Read the model definition and answer for the solid it produces. Units are mm, in the model's axes. Coordinates: 2 decimals unless noted, no trailing zeros. Write each loop counter-clockwise with the first axis right and the second up, starting at its lowest first coordinate (ties: lowest second). Pieces come first, ordered by that corner, then holes. Notation, with made-up numbers: M -32,0 L -19,0 A33 cw -19,29 Z; hole C 78.5,-14 d1. An arc over 180 degrees is marked long. Write item = value, one per line.
from build123d import *

# Parameters (mm, degrees)
BOSS_EXTRUDE2_DEPTH     = 4
SKETCH1_5_R             = 3
CUT_EXTRUDE3_DEPTH      = 54
SKETCH1_6_R             = 3
CUT_EXTRUDE4_DEPTH      = 35
CUT_EXTRUDE6_DEPTH      = 1.3
CUT_EXTRUDE6_DEPTH_BACK = 1.3


with BuildPart() as part:
    # Sketch1 → Boss-Extrude2 (new body)
    with BuildSketch(Plane(origin=(0, 0, 0), x_dir=(1, 0, 0), z_dir=(0, 1, 0))):
        with BuildLine():
            Line((-71.648984849, 27.5), (-138.40789612, 27.5))
            ThreePointArc((-138.40789612, 27.5), (-165.710949902, 25.175282852), (-192.40789612, 19))
            ThreePointArc((-192.40789612, 19), (-189.370573735, 12.036157899), (-188.40789612, 4.5))
            Line((-188.40789612, 4.5), (-120.40789612, 4.5))
            ThreePointArc((-120.40789612, 4.5), (-115.90789612, 0), (-120.40789612, -4.5))
            Line((-120.40789612, -4.5), (-188.40789612, -4.5))
            ThreePointArc((-188.40789612, -4.5), (-189.370573735, -12.036157899), (-192.40789612, -19))
            ThreePointArc((-192.40789612, -19), (-165.710949902, -25.175282852), (-138.40789612, -27.5))
            Line((-138.40789612, -27.5), (-71.648984849, -27.5))
            ThreePointArc((-71.648984849, -27.5), (65.101994969, -27.347428228), (201.798926373, -23.5))
            ThreePointArc((201.798926373, -23.5), (225.298926373, 0), (201.798926373, 23.5))
            ThreePointArc((201.798926373, 23.5), (65.101994969, 27.347428228), (-71.648984849, 27.5))
        make_face()
    extrude(amount=BOSS_EXTRUDE2_DEPTH)

    # Sketch1_5 → Cut-Extrude3 (cut)
    with BuildSketch(Plane(origin=(0, 0, 0), x_dir=(1, 0, 0), z_dir=(0, 1, 0))):
        with Locations((160.298926373, 0)):
            Circle(SKETCH1_5_R)
        with Locations((195.298926373, 0)):
            Circle(SKETCH1_5_R)
        with Locations((202.298926373, 7)):
            Circle(SKETCH1_5_R)
        with Locations((209.298926373, 0)):
            Circle(SKETCH1_5_R)
        with Locations((202.298926373, -7)):
            Circle(SKETCH1_5_R)
        with Locations((-169.40789612, -13.5)):
            Circle(SKETCH1_5_R)
    extrude(amount=CUT_EXTRUDE3_DEPTH, mode=Mode.SUBTRACT)

    # Sketch1_6 → Cut-Extrude4 (cut)
    with BuildSketch(Plane(origin=(0, 0, 0), x_dir=(1, 0, 0), z_dir=(0, 1, 0))):
        with Locations((-169.40789612, 13.5)):
            Circle(SKETCH1_6_R)
    extrude(amount=CUT_EXTRUDE4_DEPTH, mode=Mode.SUBTRACT)

    # Sketch11 → Cut-Extrude6 (cut, two sides)
    with BuildSketch(Plane(origin=(0, 2, 0), x_dir=(1, 0, 0), z_dir=(0, 1, 0))) as cut_extrude6_sk:
        with BuildLine():
            Line((-138.380243773, -23.5), (-71.624188449, -23.5))
            ThreePointArc((-71.624188449, -23.5), (56.038931481, -23.471555382), (183.66064985, -20.220401783))
            ThreePointArc((183.66064985, -20.220401783), (174.798926373, 0), (183.66064985, 20.220401783))
            ThreePointArc((183.66064985, 20.220401783), (56.038931481, 23.471555382), (-71.624188449, 23.5))
            Line((-71.624188449, 23.5), (-138.380243773, 23.5))
            ThreePointArc((-138.380243773, 23.5), (-164.744814342, 21.277783148), (-190.539098376, 15.388492851))
            ThreePointArc((-190.539098376, 15.388492851), (-191.404952918, 17.229715133), (-192.40789612, 19))
            ThreePointArc((-192.40789612, 19), (-165.710949902, 25.175282852), (-138.40789612, 27.5))
            Line((-138.40789612, 27.5), (-71.648984849, 27.5))
            ThreePointArc((-71.648984849, 27.5), (65.101994969, 27.347428228), (201.798926373, 23.5))
            ThreePointArc((201.798926373, 23.5), (225.298926373, 0), (201.798926373, -23.5))
            ThreePointArc((201.798926373, -23.5), (65.101994969, -27.347428228), (-71.648984849, -27.5))
            Line((-71.648984849, -27.5), (-138.40789612, -27.5))
            ThreePointArc((-138.40789612, -27.5), (-165.710949902, -25.175282852), (-192.40789612, -19))
            ThreePointArc((-192.40789612, -19), (-191.404952918, -17.229715133), (-190.539098376, -15.388492851))
            ThreePointArc((-190.539098376, -15.388492851), (-164.744814342, -21.277783148), (-138.380243773, -23.5))
        make_face()
    extrude(amount=CUT_EXTRUDE6_DEPTH, mode=Mode.SUBTRACT)
    extrude(cut_extrude6_sk.sketch, amount=-CUT_EXTRUDE6_DEPTH_BACK, mode=Mode.SUBTRACT)


solid = part.part
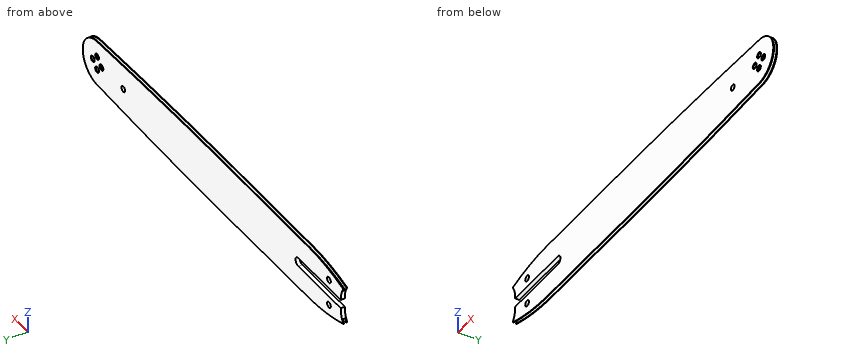
Item 1: Flat-ended cylindrical pins translate along their axes: pin 1 (1 mm diameter, centred on x = 169, y = 3, fed in from -Z); pin 2 (5 mm diameter, centred on x = 195.3, z = 0, fed in from -Y); pin 3 (0.8 mm diameter, centred on x = -111, y = 2.5, fed in from +Z); pin 4 (0.8 mm diameter, centred on x = -94, y = 3.5, fed in from -Z). Find the tip coordinate at first contact, or state that the pin passes through.
Worked answers:
pin_1 = -24.77
pin_2 = through
pin_3 = 23.5
pin_4 = -27.5
Item 2: Find section A-A (y = 2.3). Determine the outline of the cut face in (x, z).
Worked answers:
outline = M -190.54,-15.39 A188.63 ccw -138.38,-23.5 L -71.62,-23.5 A5056.78 ccw 183.66,-20.22 A27.5 cw 183.66,20.22 A5056.78 ccw -71.62,23.5 L -138.38,23.5 A188.63 ccw -190.54,15.39 A26.82 cw -188.41,4.5 L -120.41,4.5 A4.5 cw -120.41,-4.5 L -188.41,-4.5 A26.82 cw Z; hole C -169.41,-13.5 d6; hole C -169.41,13.5 d6; hole C 160.3,0 d6
Item 3: Find section B-B (x = -163). Determine the outline of the cut face in (y, z).
Worked answers:
outline = M 0,-25.58 L 0.7,-25.58 L 0.7,-21.54 L 3.3,-21.54 L 3.3,-25.58 L 4,-25.58 L 4,-4.5 L 0,-4.5 Z; M 0,4.5 L 4,4.5 L 4,25.58 L 3.3,25.58 L 3.3,21.54 L 0.7,21.54 L 0.7,25.58 L 0,25.58 Z
Item 4: Consider line 1 along Y through (x, z) = (137, 24.5); line 2 along Z through (x, y) = (-125, 1.65); line 3 along Z through (x, y) = (-105.5, 0.4). Determine where each line is inside the solid, lowest interval first. Write a range as from..to.
Worked answers:
line_1 = 0..0.7, 3.3..4
line_2 = -23.5..-4.5, 4.5..23.5
line_3 = -27.5..27.5
